Design review of the part shown in the three views and the two pictorial views. Dimensions are in mm from the part's minimum x, y and z. Coordinates: 2 decimals unless noted, no trailing zeros. Write each loop counter-clockwise with the first axis right and the second up, starting at its lowest first coordinate (ties: lowest second). Pieces come first, ordered by that corner, then holes. Notation, with made-up numbers: M 13,-6.5 L 40,-6.5 A23 cw 40,28.5 Z; hole C 67.25,-7 d1. An arc over 180 degrees is marked long. Answer as a JSON object with one key per item and string values.
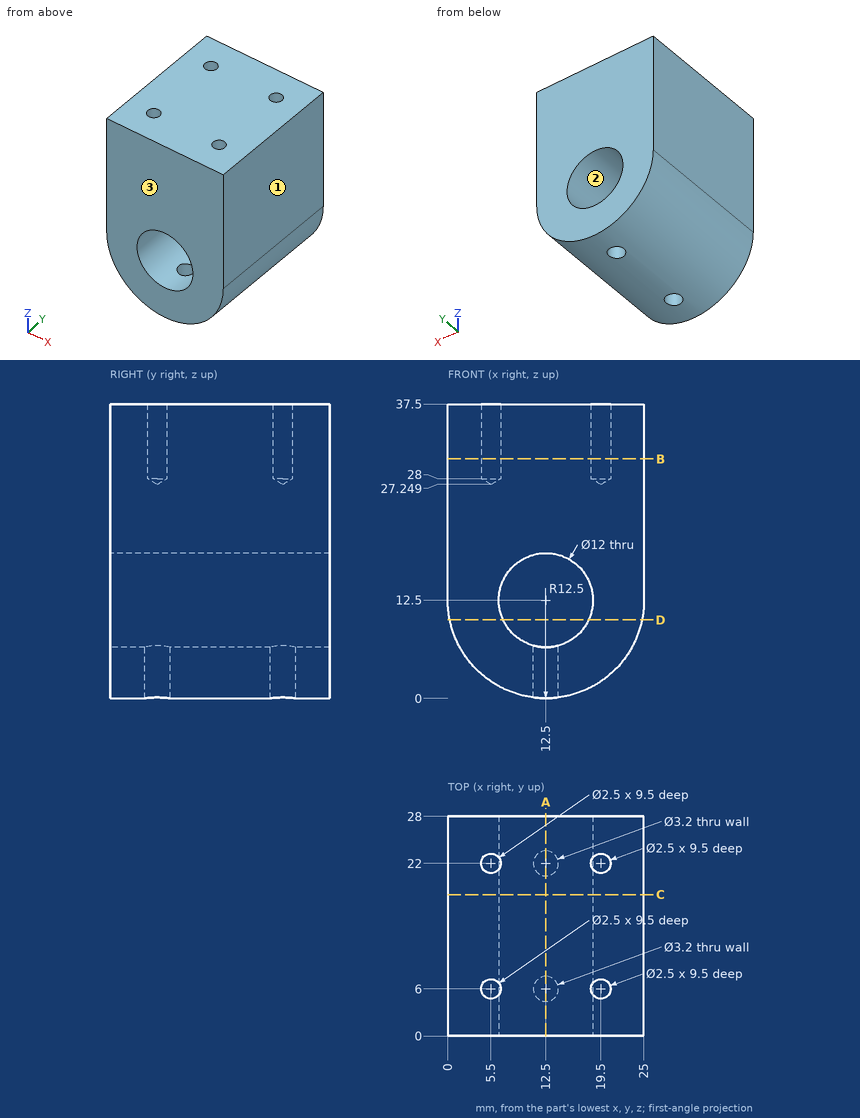
(1) For pin 1 Ø1.5 at (y, z) = (21.5, 5.5) entering from +X; pin 2 Ø8 at (x, y) = (6, 16.5) entering from -Z; pin 3 Ø2 at (x, y) = (19, 24) entering from -Z (3 decimals), all flat-tipped, find the tip position at first contact; note any pin that passes through.
Results list:
{"pin 1": "x = 23.33", "pin 2": "z = 0.25", "pin 3": "z = 1.275"}
(2) Add section B-B on z = 30.5. Give the boundary of the cut face in (x, y).
Results list:
{"outline": "M 0,0 L 25,0 L 25,28 L 0,28 Z; hole C 5.5,6 d2.5; hole C 5.5,22 d2.5; hole C 19.5,6 d2.5; hole C 19.5,22 d2.5"}
(3) Add section C-C on y = 18. Give the boundary of the cut face in (x, z).
Results list:
{"outline": "M 0,12.5 A12.5 ccw 25,12.5 L 25,37.5 L 0,37.5 Z; hole C 12.5,12.5 d12"}
(4) Draft analysis for pull direction X (two halves, no side actions). For the marked faces 1, 2 and 3, state which applies: released by +X, released by -X, zero draft, split by the parting line, or undercut.
Results list:
{"face 1": "released by +X", "face 2": "undercut", "face 3": "zero draft"}
(5) Add section D-D on z = 10. Give the boundary of the cut face in (x, y).
Results list:
{"outline": "M 0.25,0 L 7.05,0 L 7.05,28 L 0.25,28 Z; M 17.95,0 L 24.75,0 L 24.75,28 L 17.95,28 Z"}
(6) Wall thickness on line 1 along Y through (x, z) = (5.5, 35.25); line 2 along X through (y, z) = (21, 29.5); line 3 along Z through (x, y) = (12.25, 20): over which ranges is each line inside the solid? List them lowest first. Write a range as from..to.
Results list:
{"line 1": "0..4.75, 7.25..20.75, 23.25..28", "line 2": "0..4.75, 6.25..18.75, 20.25..25", "line 3": "0..6.51, 18.49..37.5"}
(7) Add section A-A on x = 12.5. Give the boundary of the cut face in (y, z).
Results list:
{"outline": "M 0,0 L 4.4,0 L 4.4,6.5 L 0,6.5 Z; M 0,18.5 L 28,18.5 L 28,37.5 L 0,37.5 Z; M 7.6,0 L 20.4,0 L 20.4,6.5 L 7.6,6.5 Z; M 23.6,0 L 28,0 L 28,6.5 L 23.6,6.5 Z"}
